from build123d import *

# Parameters (mm, degrees)
SKETCH1_R           = 50.292
SKETCH1_R_2         = 3.475
BOSS_EXTRUDE1_DEPTH = 5


with BuildPart() as part:
    # Sketch1 → Boss-Extrude1 (new body)
    with BuildSketch(Plane(origin=(0, 0, 0), x_dir=(1, 0, 0), z_dir=(0, 1, 0))):
        Circle(SKETCH1_R)
        with Locations((42.886820356, 1.924977859)):
            Circle(SKETCH1_R_2, mode=Mode.SUBTRACT)
        with Locations((-42.886820356, 1.924977859)):
            Circle(SKETCH1_R_2, mode=Mode.SUBTRACT)
        with Locations((-37.000474826, -12.718618748)):
            Circle(SKETCH1_R_2, mode=Mode.SUBTRACT)
        with Locations((-23.129730363, 31.556520301)):
            Circle(SKETCH1_R_2, mode=Mode.SUBTRACT)
        with Locations((37.000474826, -12.718618748)):
            Circle(SKETCH1_R_2, mode=Mode.SUBTRACT)
        with Locations((23.129730363, 31.556520301)):
            Circle(SKETCH1_R_2, mode=Mode.SUBTRACT)
    extrude(amount=BOSS_EXTRUDE1_DEPTH)


solid = part.part
Could you check a few things on this model? Use its own coordinates, in mm. Coordinates: 2 decimals unless noted, no trailing zeros. Order: outer loops, then holes, each group sorted by start corner. A loop starts at its lowest first (then second) coordinate and runs counter-clockwise, first axis right, second up. Notation, with made-up numbers: (-7, 24.5) - (5, 24.5) arc R31 cw to (5, 53.5) - close; hole circle Ø10 at (-15.75, 23). An arc over 180 degrees is marked (long way). Answer in a Markdown table with one row per item. Add a question column.
(1) I need wall thicknesses on L1, parallel to X at y = 0.3, z = -34.5; L2, parallel to Z at x = 1.5, y = 3.7; L3, parallel to X at y = 4.1, z = 19.5. Which ranges of each line are inside material? Lowest first, please.
(2) Will this pin go through, and if not, where does the flat tip stop? pin 1 (2 mm diameter, centred on y = 0.5, z = -32.5, fed in from -X).
(3) If we section it at A-A, the plane y = 2.8: Please give me the cut outline in (x, z) (3 decimals), then the cut area to 3 significant figures.
(4) If we mould it in two halves opening along Z, with no side actions, what happens to faces 1 (the face through (-10.902, 2.465, 49.096)), 2 (the face through (-1, 5, -1)), 3 (the face through (-19.815, 2.465, -32.6))? For each: released by +Z, released by -Z, zero draft, split by the parting line, or undercut.
(5) If we section it at D-D, the plane z = 39.5: Please give me the cut outline in (x, y).
(6) If we section it at C-C, the plane x = 24: Please give me the cut outline in (y, z), then the cut area to 3 significant figures.
(7) If we section it at B-B, the plane z = 0: Please give me the cut outline in (x, y), then the cut area to 3 significant figures.
Results are:
| question | item | result |
|---|---|---|
| 1 | L1 | x = -36.59 to -24.98, -21.28 to 21.28, 24.98 to 36.59 |
| 1 | L2 | z = -50.27 to 50.27 |
| 1 | L3 | x = -46.36 to 46.36 |
| 2 | pin 1 | stops at x = -39.21 |
| 3 | outline | circle Ø100.584 at (0, 0); hole circle Ø6.95 at (-42.887, -1.925); hole circle Ø6.95 at (-37, 12.719); hole circle Ø6.95 at (-23.13, -31.557); hole circle Ø6.95 at (23.13, -31.557); hole circle Ø6.95 at (37, 12.719); hole circle Ø6.95 at (42.887, -1.925) |
| 3 | area | 7,720 mm2 |
| 4 | face 1 | split by the parting line |
| 4 | face 2 | zero draft |
| 4 | face 3 | undercut |
| 5 | outline | (-31.13, 0) - (31.13, 0) - (31.13, 5) - (-31.13, 5) - close |
| 6 | outline | (0, -44.2) - (5, -44.2) - (5, -34.92) - (0, -34.92) - close; (0, -28.19) - (5, -28.19) - (5, 44.2) - (0, 44.2) - close |
| 6 | area | 408 mm2 |
| 7 | outline | (-50.29, 0) - (-45.78, 0) - (-45.78, 5) - (-50.29, 5) - close; (-39.99, 0) - (39.99, 0) - (39.99, 5) - (-39.99, 5) - close; (45.78, 0) - (50.29, 0) - (50.29, 5) - (45.78, 5) - close |
| 7 | area | 445 mm2 |
